Source: three-view drawing plus pictorial views. Frame: mm from the lowest corner of the part. A direction names the side the tool comes from. Give positions to 0.01 mm unless a question says otherwise; leave off trailing zeros. Write each loop counter-clockwise with the first axis right and the second up, starting at its lowest first coordinate (ties: lowest second). Pieces come first, ordered by that corner, then holes. Notation, with made-up numbers: (39, -36) - (52, -36) arc R31 cw to (52, -10) - close; hole circle Ø5 at (-24, 87). An arc over 180 degrees is marked (long way). One line per question, with ' | ' between items. Start each with the question number.
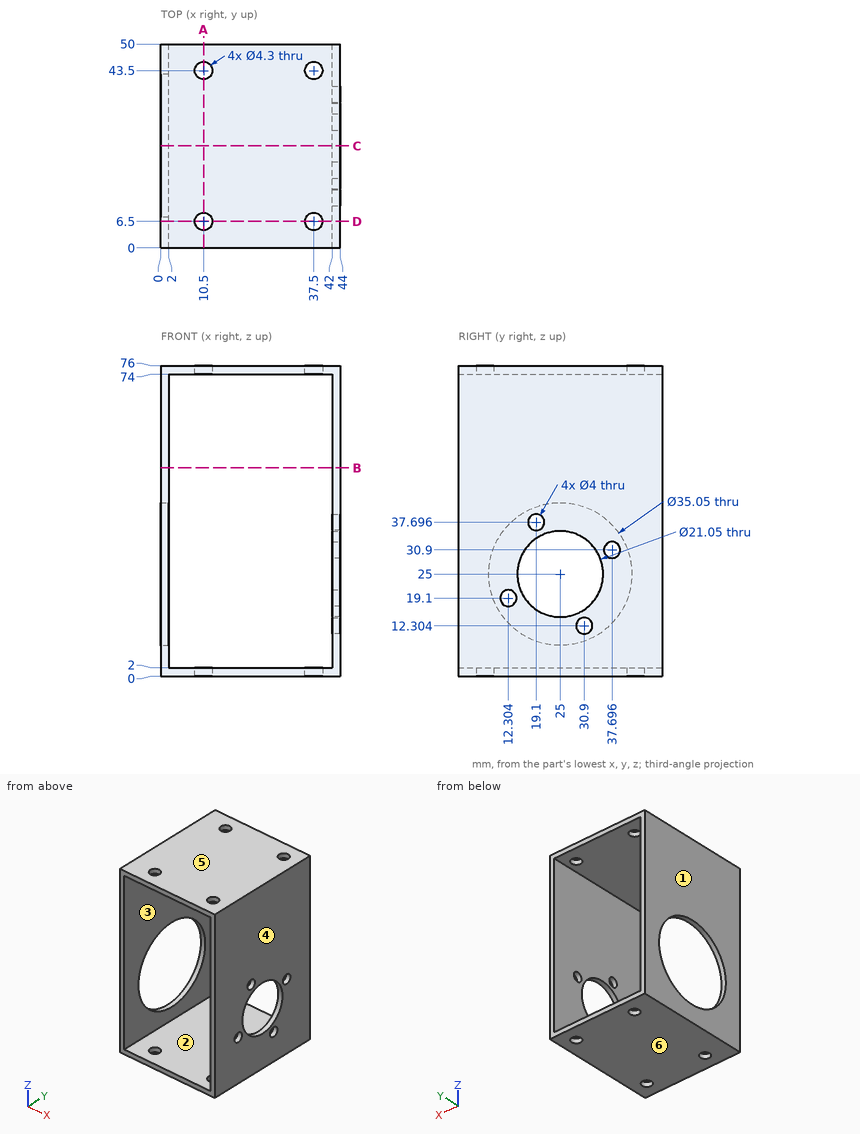
1) Pull-direction query (Z, two-part tool) for the marked faces 3, 4, 5 and 6; classes: +Z half, -Z half, draft (parallel to the pull), parting line (faces both ways), or undercut.
2) Section D-D, the plane y = 6.5. Output: boundary loops of the cut face in (x, z), plus the area to 3 significant figures.
3) First-contact query: pin 1 Ø17 at (y, z) = (25, 25) entering from -X; pin 2 Ø1.5 at (y, z) = (21, 41) entering from -X. Flat tips, straight axial feed; report the tip coordinate or a pass-through.
4) Reachability of the marked faces 1 and 2 from +Z, -Z, +X, -X, +Y, -Y: full face, straight path, thin tool, end or side. Return the list, or none.
5) Section A-A, the plane x = 10.5. Output: boundary loops of the cut face in (y, z), plus the area to 3 significant figures.
6) Section C-C, the plane y = 25. Output: boundary loops of the cut face in (x, z) (3 decimals).
7) Section B-B, the plane z = 51. Output: boundary loops of the cut face in (x, y).
8) Line query: L1, parallel to Y at x = 10.5, z = 75.05; L2, parallel to Z at x = 13, y = 8; L3, parallel to X at y = 11, z = 61.5. Output: solid intervals per line, ascending.
Answer key:
1) face 3: undercut | face 4: draft | face 5: +Z half | face 6: -Z half
2) outline: (0, 0) - (8.35, 0) - (8.35, 2) - (2, 2) - (2, 74) - (8.35, 74) - (8.35, 76) - (0, 76) - close; (12.65, 0) - (35.35, 0) - (35.35, 2) - (12.65, 2) - close; (12.65, 74) - (35.35, 74) - (35.35, 76) - (12.65, 76) - close; (39.65, 0) - (44, 0) - (44, 76) - (39.65, 76) - (39.65, 74) - (42, 74) - (42, 2) - (39.65, 2) - close | area: 430 mm^2
3) pin 1: through | pin 2: x = 42
4) face 1: +Z, -Z, -X, +Y, -Y | face 2: +Y, -Y
5) outline: (0, 0) - (4.35, 0) - (4.35, 2) - (0, 2) - close; (0, 74) - (4.35, 74) - (4.35, 76) - (0, 76) - close; (8.65, 0) - (41.35, 0) - (41.35, 2) - (8.65, 2) - close; (8.65, 74) - (41.35, 74) - (41.35, 76) - (8.65, 76) - close; (45.65, 0) - (50, 0) - (50, 2) - (45.65, 2) - close; (45.65, 74) - (50, 74) - (50, 76) - (45.65, 76) - close | area: 166 mm^2
6) outline: (0, 0) - (44, 0) - (44, 14.475) - (42, 14.475) - (42, 2) - (2, 2) - (2, 7.475) - (0, 7.475) - close; (0, 42.525) - (2, 42.525) - (2, 74) - (42, 74) - (42, 35.525) - (44, 35.525) - (44, 76) - (0, 76) - close
7) outline: (0, 0) - (2, 0) - (2, 50) - (0, 50) - close; (42, 0) - (44, 0) - (44, 50) - (42, 50) - close
8) L1: 0 to 4.35, 8.65 to 41.35, 45.65 to 50 | L2: 0 to 2, 74 to 76 | L3: 0 to 2, 42 to 44
